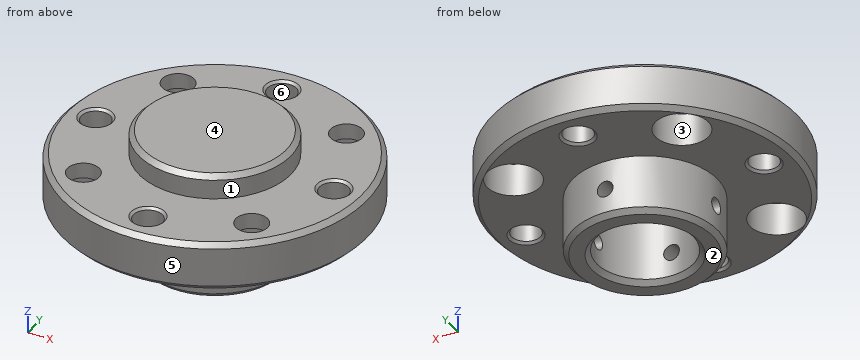
```python
from build123d import *

# Parameters (mm, degrees)
SKETCH_2_R               = 3.3
SKETCH_2_R_2             = 3
CUT_EXTRUDE_1_DEPTH      = 10
SKETCH_2_3_R             = 5.5
SKETCH_2_3_R_2           = 3.3
CUT_EXTRUDE_2_DEPTH      = 6.8
CHAMFER_1_SIZE           = 1
CHAMFER_2_SIZE           = 1
CHAMFER_3_SIZE           = 1
SKETCH_5_W               = 1.65
SKETCH_5_H               = 31.5
PATTERN_CIRCULAR_1_COUNT = 4
CHAMFER_4_SIZE           = 0.5
CHAMFER_5_SIZE           = 1


with BuildPart() as part:
    # 草图1 → 旋转1 (revolve)
    with BuildSketch(Plane(origin=(0, 0, 0), x_dir=(0, 0, -1), z_dir=(1, 0, 0)), mode=Mode.PRIVATE) as revolve_1_sk:
        Polygon((0, 0), (0, 15.75), (5, 15.75), (5, 31.5), (15, 31.5), (15, 15), (27, 15), (27, 10), (3, 10), (3, 0), align=None)
    revolve(revolve_1_sk.sketch.rotate(Axis((0, 0, 27.099264706), (0, 0, -1)), 90), axis=Axis((0, 0, 27.099264706), (0, 0, -1)))

    # 草图2 → 切除-拉伸1 (cut)
    with BuildSketch(Plane(origin=(0, 0, -15), x_dir=(-1, 0, 0), z_dir=(0, 0, -1))):
        with Locations((-17.67766953, 17.67766953)):
            Circle(SKETCH_2_R)
        with Locations((0, 25)):
            Circle(SKETCH_2_R_2)
        with Locations(Location((17.67766953, 17.67766953, 0), (0, 0, 180))):
            Circle(SKETCH_2_R)
        with Locations((17.67766953, -17.67766953)):
            Circle(SKETCH_2_R)
        with Locations(Location((-17.67766953, -17.67766953, 0), (0, 0, 180))):
            Circle(SKETCH_2_R)
        with Locations(Location((0, -25, 0), (0, 0, 180))):
            Circle(SKETCH_2_R_2)
        with Locations(Location((-25, 0, 0), (0, 0, 180))):
            Circle(SKETCH_2_R_2)
        with Locations((25, 0)):
            Circle(SKETCH_2_R_2)
    extrude(amount=-CUT_EXTRUDE_1_DEPTH, mode=Mode.SUBTRACT)

    # 草图2<3> → 切除-拉伸2 (cut)
    # profile 1 of 4: a face of its own
    with BuildSketch(Plane(origin=(0, 0, -15), x_dir=(-1, 0, 0), z_dir=(0, 0, -1))):
        with Locations((-17.67766953, 17.67766953)):
            Circle(SKETCH_2_3_R)
        with Locations((-17.67766953, 17.67766953)):
            Circle(SKETCH_2_3_R_2, mode=Mode.SUBTRACT)
    # profile 2 of 4: a face of its own
    with BuildSketch(Plane(origin=(0, 0, -15), x_dir=(-1, 0, 0), z_dir=(0, 0, -1))):
        with Locations((17.67766953, 17.67766953)):
            Circle(SKETCH_2_3_R)
        with Locations((17.67766953, 17.67766953)):
            Circle(SKETCH_2_3_R_2, mode=Mode.SUBTRACT)
    # profile 3 of 4: a face of its own
    with BuildSketch(Plane(origin=(0, 0, -15), x_dir=(-1, 0, 0), z_dir=(0, 0, -1))):
        with Locations((17.67766953, -17.67766953)):
            Circle(SKETCH_2_3_R)
        with Locations((17.67766953, -17.67766953)):
            Circle(SKETCH_2_3_R_2, mode=Mode.SUBTRACT)
    # profile 4 of 4: a face of its own
    with BuildSketch(Plane(origin=(0, 0, -15), x_dir=(-1, 0, 0), z_dir=(0, 0, -1))):
        with Locations((-17.67766953, -17.67766953)):
            Circle(SKETCH_2_3_R)
        with Locations((-17.67766953, -17.67766953)):
            Circle(SKETCH_2_3_R_2, mode=Mode.SUBTRACT)
    extrude(amount=-CUT_EXTRUDE_2_DEPTH, mode=Mode.SUBTRACT)

    # 倒角1
    chamfer_1_edges = [part.edges().sort_by_distance(p)[0] for p in [
        (-15.75, 0, 0),
    ]]
    chamfer(chamfer_1_edges, length=CHAMFER_1_SIZE)

    # 倒角2
    chamfer_2_edges = [part.edges().sort_by_distance(p)[0] for p in [
        (-10, 0, -27),
    ]]
    chamfer(chamfer_2_edges, length=CHAMFER_2_SIZE)

    # 倒角3
    chamfer_3_edges = [part.edges().sort_by_distance(p)[0] for p in [
        (-31.5, 0, -15),
        (-31.5, 0, -5),
    ]]
    chamfer(chamfer_3_edges, length=CHAMFER_3_SIZE - 0.0001)  # a hair under: the kernel refuses the full size

    # 草图5 → M4 螺纹孔1 (revolve, cut)
    with BuildSketch(Plane(origin=(0, 0, -21), x_dir=(0, 0, -1), z_dir=(1, 0, 0))):
        with Locations((0.825, 15.75)):
            Rectangle(SKETCH_5_W, SKETCH_5_H)
    hole_wizard_m4_1 = revolve(axis=Axis((0, -6.35, -21), (0, 1, 0)), mode=Mode.SUBTRACT)

    # 阵列(圆周)1: M4 螺纹孔1 ×4 about axis
    pattern_circular_1_axis = Axis((0, 0, -27), (0, 0, 1))
    for i in range(1, PATTERN_CIRCULAR_1_COUNT):
        add(hole_wizard_m4_1.rotate(pattern_circular_1_axis, i * 360 / PATTERN_CIRCULAR_1_COUNT), mode=Mode.SUBTRACT)

    # 倒角4
    chamfer_4_edges = [part.edges().sort_by_distance(p)[0] for p in [
        (22, 0, -15),
        (22, 0, -5),
        (3, 25, -5),
        (3, 25, -15),
        (-22, 0, -5),
        (-22, 0, -15),
        (-3, -25, -15),
        (-3, -25, -5),
    ]]
    chamfer(chamfer_4_edges, length=CHAMFER_4_SIZE)

    # 倒角5
    chamfer_5_edges = [part.edges().sort_by_distance(p)[0] for p in [
        (-15, 0, -27),
    ]]
    chamfer(chamfer_5_edges, length=CHAMFER_5_SIZE)


solid = part.part
```
Can you work these out from the model? Positions are in its coordinate system, mm. Face numbers are marked on the shaded views. A direction names the side the tool comes from. Round coordinates to 2 decimals unless told otherwise and drop trailing zeros. Loops run counter-clockwise (first coordinate to the right, second up) from the corner with the lowest first, then second, coordinate; pieces in that order, holes last.
Item 1: Suppose I cut it at A-A, the plane z = -21. Write out the boundary of the cut face in (x, y).
Item 2: Please list where these lines run through material, in increasing order: L1, parallel to X at y = -20, z = -10.5; L2, parallel to X at y = 0.5, z = -10.5; L3, parallel to Z at x = 0, y = 13.
Item 3: Suppose I cut it at B-B, the plane y = 0. State how many separate pieces and enclosed holes the cut face has, then the cut area to 4 significant figures.
Item 4: Which directions (+Z, -Z, +X, -X, +Y, -Y) give clear straight access to the entire face, cutting with the end or side of a thin tool? Please do the marked faces 1, 2 and 3.
Item 5: Will these pins go through, and if not, where does the flat tip stop? pin 1 Ø5.5 at (x, y) = (0, 25) entering from +Z; pin 2 Ø8.5 at (x, y) = (-17.68, 17.68) entering from +Z; pin 3 Ø6 at (x, z) = (9, -15.5) entering from -Y; pin 4 Ø12 at (y, z) = (-18, -5.5) entering from +X.
Item 6: If we mould it in two halves opening along Y, with no side actions, what happens to the marked faces 4, 5 and 6? For each: +Y half, -Y half, draft (parallel to the pull), parting line (faces both ways), or undercut.
Reported:
1. outline: (-14.91, -1.65) arc R15 ccw to (-1.65, -14.91) - (-1.65, -9.86) arc R10 cw to (-9.86, -1.65) - close; (-14.91, 1.65) - (-9.86, 1.65) arc R10 cw to (-1.65, 9.86) - (-1.65, 14.91) arc R15 ccw to start; (1.65, -14.91) arc R15 ccw to (14.91, -1.65) - (9.86, -1.65) arc R10 cw to (1.65, -9.86) - close; (1.65, 9.86) arc R10 cw to (9.86, 1.65) - (14.91, 1.65) arc R15 ccw to (1.65, 14.91) - close
2. L1: x = -24.34 to -22.66, -12.69 to 12.69, 22.66 to 24.34
2. L2: x = -31.5 to -27.96, -22.04 to -9.99, 9.99 to 22.04, 27.96 to 31.5
2. L3: z = -27 to -22.65, -19.35 to 0
3. separate pieces: 5
3. enclosed holes: 0
3. area: 508.5 mm2
4. face 1: +Z
4. face 2: -Z, +X, -X, +Y, -Y
4. face 3: -Z
5. pin 1: passes through
5. pin 2: stops at z = -5
5. pin 3: stops at y = -30.84
5. pin 4: stops at x = 29.12
6. face 4: draft
6. face 5: parting line
6. face 6: undercut
